Work out the finished part from the listing and answer in its coordinate system (mm). Coordinates: 2 decimals unless noted, no trailing zeros. Order: outer loops, then holes, each group sorted by start corner. A loop starts at its lowest first (then second) coordinate and runs counter-clockwise, first axis right, second up. Notation, with made-up numbers: M 54.5,89.25 L 84.5,89.25 A18 cw 84.5,113.25 Z; hole C 72.25,18.5 d5. An arc over 180 degrees is marked long. Write item = value, one per line. Start each with the question number.
Q1. Find section A-A on y = -542.5. Give the vertices of the cut face in (x, z).
Q2. A straight line is drawn through the part: line 1 along Y through (x, z) = (907.5, -412.5). Find the intervals that lie inside material, in ascending order.
Q3. Find section B-B on z = -390.5. Give the vertices of the cut face in (x, y), and give its area (3 significant figures).
Q4. Find section C-C on x = 963. Give the vertices of the cut face in (y, z), and give its area (3 significant figures).
Q5. Each of these flat-tipped pins is pushed along its axis until it touches: P1, Ø10, axis at x = 237.5, z = -283, coming from the -Y side; P2, Ø9, axis at x = 1179, y = -483.5, coming from the +Z side. Where does it stop, or does it pass through?
Autodesk Fusion 360 part; units mm, degrees
sketch "Sketch1" plane through (0, 0, 0) normal (0, 1, 0) x (1, 0, 0)
  line L0 (0, 0) -> (1200, 0)
  line L1 (1200, 0) -> (1200, 600)
  line L2 (1200, 600) -> (0, 600)
  line L3 (0, 600) -> (0, 0)
extrude "Extrude1" add sketch "Sketch1" along normal blind 30
sketch "Sketch2" plane through (0, 0, 0) normal (0, -1, 0) x (1, 0, 0)
  line L0 (0, 0) -> (0, -600)
  line L1 (0, -600) -> (1200, -600)
  line L2 (1200, -600) -> (1200, 0)
  line L3 (1200, 0) -> (0, 0)
  line L4 (0, 0) -> (30, 0)
  line L5 (30, 0) -> (30, -30)
  line L6 (30, -30) -> (0, -30)
  line L7 (0, -30) -> (0, 0)
  line L8 (0, -600) -> (30, -600)
  line L9 (30, -600) -> (30, -570)
  line L10 (30, -570) -> (0, -570)
  line L11 (0, -570) -> (0, -600)
  line L12 (1200, 0) -> (1170, 0)
  line L13 (1170, 0) -> (1170, -30)
  line L14 (1170, -30) -> (1200, -30)
  line L15 (1200, -30) -> (1200, 0)
  line L16 (1200, -600) -> (1170, -600)
  line L17 (1170, -600) -> (1170, -570)
  line L18 (1170, -570) -> (1200, -570)
  line L19 (1200, -570) -> (1200, -600)
extrude "Extrude2" add sketch "Sketch2" along normal blind 730 contours L0 L3 L4 L5 L6 L7 | L0 L1 L8 L9 L10 L11 | L2 L3 L12 L13 L14 L15 | L1 L2 L16 L17 L18 L19
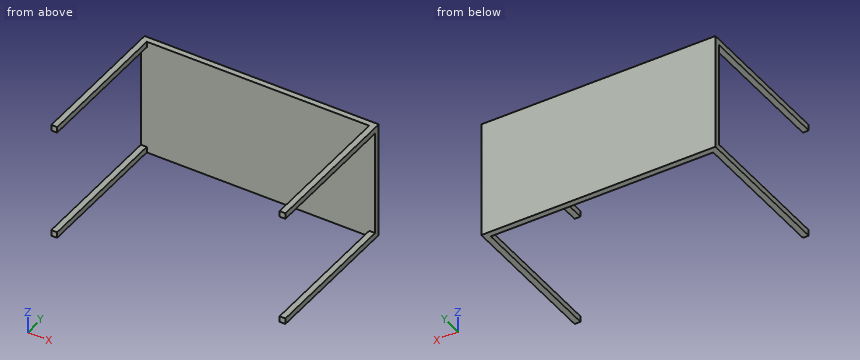
Findings below:
q1.outline = M 0,-600 L 30,-600 L 30,-570 L 0,-570 Z; M 0,-30 L 30,-30 L 30,0 L 0,0 Z; M 1170,-600 L 1200,-600 L 1200,-570 L 1170,-570 Z; M 1170,-30 L 1200,-30 L 1200,0 L 1170,0 Z
q2.line_1 = 0 to 30
q3.outline = M 0,0 L 1200,0 L 1200,30 L 0,30 Z
q3.area = 36,000 mm^2
q4.outline = M 0,-600 L 30,-600 L 30,0 L 0,0 Z
q4.area = 18,000 mm^2
q5.P1 = 0
q5.P2 = 0
